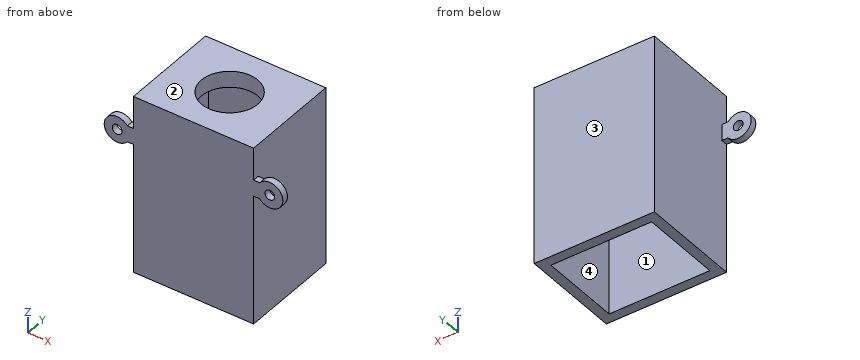
Autodesk Fusion 360 part; units mm, degrees
sketch "Sketch1" plane through (0, 0, 0) normal (0, 0, 1) x (1, 0, 0)
  line L0 (0, 50) -> (37, 50)
  line L1 (37, 50) -> (37, 19)
  line L2 (37, 19) -> (0, 19)
  line L3 (0, 19) -> (0, 50)
  line L4 (3, 22) -> (3, 47)
  line L5 (3, 47) -> (34, 47)
  line L6 (34, 47) -> (34, 22)
  line L7 (34, 22) -> (3, 22)
  dimension "d1" = 37
  dimension "d2" = 31
  dimension "d3" = 3
extrude "Extrude1" add sketch "Sketch1" along normal blind 55
sketch "Sketch2" plane through (0, 0, 55) normal (0, 0, 1) x (-1, 0, 0)
  line L0 (-34, -47) -> (-34, -22)
  line L1 (-34, -22) -> (-3, -22)
  line L2 (-3, -22) -> (-3, -47)
  line L3 (-3, -47) -> (-34, -47)
  line L4 (0, -19) -> (-37, -19)
  line L5 (-37, -19) -> (-37, -50)
  line L6 (-37, -50) -> (0, -50)
  line L7 (0, -50) -> (0, -19)
  line L8 (0, -50) -> (-37, -50)
  line L9 (-37, -50) -> (-37, -19)
  line L10 (-37, -19) -> (0, -19)
  line L11 (0, -19) -> (0, -50)
  circle A0 centre (-18.5, -34.5) radius 8.6861
extrude "Extrude2" add sketch "Sketch2" against normal blind 5 contours L0 L1 L2 L3 | L4 L5 L6 L7 L8 L9 L10 L11
sketch "Sketch3" plane through (0, 19, 0) normal (0, -1, 0) x (1, 0, 0)
  line L0 (0, 55) -> (0, 0)
  line L1 (0, 0) -> (37, 0)
  line L2 (37, 0) -> (37, 55)
  line L3 (37, 55) -> (0, 55)
  line L4 (0, 40) -> (-5, 40)
  line L5 (-5, 40) -> (-5, 45)
  line L6 (-5, 45) -> (0, 45)
  line L7 (0, 45) -> (0, 40)
  line L8 (37, 40) -> (42, 40)
  line L9 (42, 40) -> (42, 45)
  line L10 (42, 45) -> (37, 45)
  circle A0 centre (-5, 42.5) radius 1.5
  circle A1 centre (-5, 42.5) radius 4
  circle A2 centre (42, 42.5) radius 1.5
  circle A3 centre (42, 42.5) radius 4
  line L11 (35, 40) -> (38, 40)
  line L12 (38, 40) -> (38, 45)
  line L13 (38, 45) -> (35, 45)
  line L14 (1.6164, 40) -> (-1, 40)
  line L15 (-1, 40) -> (-1, 45)
  line L16 (-1, 45) -> (1.6164, 45)
  line L17 (35, 40) -> (35, 45)
  line L18 (1.6164, 40) -> (1.6164, 45)
  dimension "d9" = 5
  dimension "d10" = 3
  dimension "d11" = 2.5
  dimension "d12" = 3
  dimension "d13" = 2.5
extrude "Extrude3" add sketch "Sketch3" against normal blind 2 contours L0 L7 L14 L16 L18 | L0 L4 L6 L7 L14 L15 L16 | L6 A1 L15 | L2 L8 L10 L11 L12 L13 | L2 L11 L13 L17 | L4 A1 L15 | L4 L5 L6 A0 A1 | L4 L5 L6 A0 A1 | L10 A3 L12 | L8 A3 L12 | L8 L9 L10 A2 A3 | L8 L9 L10 A2 A3
Geometry check sheet. Reference: the model listing, model coordinates, mm. Face numbers are marked on the shaded views. A direction names the side the tool comes from. Give positions to 0.01 mm unless a question says otherwise; leave off trailing zeros. Loops run counter-clockwise (first coordinate to the right, second up) from the corner with the lowest first, then second, coordinate; pieces in that order, holes last. Notation, with made-up numbers: M -20.5,83 L -3.5,83 A27 ccw -3.5,114 Z; hole C 29,1 d11. An arc over 180 degrees is marked long. Answer as a JSON object with one key per item and string values. Group by question number.
Item 1: Mould release check, pull along X, two halves, no side actions. Record for the marked faces 3 and 4: pulls with the +X half, pulls with the -X half, needs draft (parallel to the pull), parting line crosses it, or undercut.
Item 2: Sectioned sample at A-A on z = 42.5. Record the boundary of the cut face in (x, y), plus the area to 3 significant figures.
Item 3: Gauge pin test, flat ends, axial feed: pin 1 (7.5 mm diameter, centred on y = 30.5, z = 24, fed in from -X); pin 2 (2 mm diameter, centred on x = 23.5, y = 30, fed in from +Z); pin 3 (2.5 mm diameter, centred on x = 40.5, z = 41.5, fed in from +Y); pin 4 (1.5 mm diameter, centred on x = -1, y = 20.5, fed in from +Z). Record the tip position at first contact, or that the pin passes through.
Item 4: Sectioned sample at B-B on x = 18.5. Record the boundary of the cut face in (y, z), plus the area to 3 significant figures.
Item 5: Material ranges on L1, parallel to X at y = 19.75, z = 42.5; L2, parallel to Z at x = -5, y = 20; L3, parallel to X at y = 34.5, z = 53.15, recorded low to high.
Item 6: Access from +Z, -Z, +X, -X, +Y, -Y to the whole of each face (thin tool, end or side, straight path). Record for the marked faces 1 and 2.
Item 7: Sectioned sample at C-C on z = 7. Record the boundary of the cut face in (x, y).
Item 8: Sectioned sample at D-D on y = 34.5. Record the boundary of the cut face in (x, z).
Findings below:
{
 "1": {"face 3": "needs draft", "face 4": "undercut"},
 "2": {"outline": "M -9,19 L -6.5,19 L -6.5,21 L -9,21 Z; M -3.5,19 L 40.5,19 L 40.5,21 L 37,21 L 37,50 L 0,50 L 0,21 L -3.5,21 Z; M 43.5,19 L 46,19 L 46,21 L 43.5,21 Z; hole M 3,22 L 34,22 L 34,47 L 3,47 Z", "area": "396 mm2"},
 "3": {"pin 1": "x = 0", "pin 2": "through", "pin 3": "y = 21", "pin 4": "z = 45"},
 "4": {"outline": "M 19,0 L 22,0 L 22,50 L 25.81,50 L 25.81,55 L 19,55 Z; M 43.19,50 L 47,50 L 47,0 L 50,0 L 50,55 L 43.19,55 Z", "area": "368 mm2"},
 "5": {"L1": "-9 to -6.5, -3.5 to 40.5, 43.5 to 46", "L2": "38.5 to 41, 44 to 46.5", "L3": "0 to 9.81, 27.19 to 37"},
 "6": {"face 1": "-Z", "face 2": "+Z, +X, -X, +Y, -Y"},
 "7": {"outline": "M 0,19 L 37,19 L 37,50 L 0,50 Z; hole M 3,22 L 34,22 L 34,47 L 3,47 Z"},
 "8": {"outline": "M 0,0 L 3,0 L 3,50 L 9.81,50 L 9.81,55 L 0,55 Z; M 27.19,50 L 34,50 L 34,0 L 37,0 L 37,55 L 27.19,55 Z"}
}
